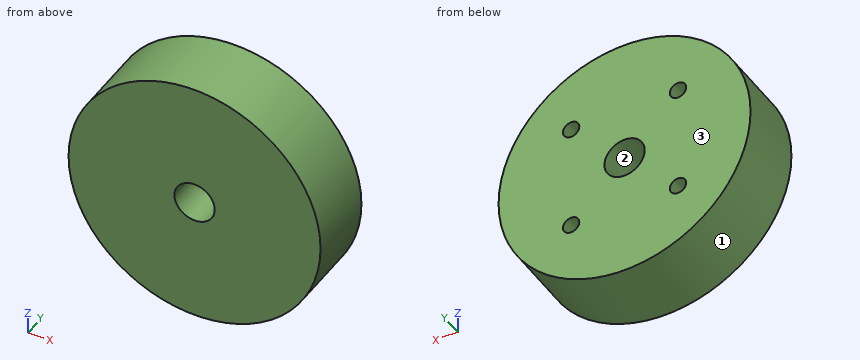
Autodesk Inventor part; units mm, degrees
ref_plane "YZ Plane" through (0, 0, 0) normal (1, 0, 0) x (0, 1, 0)
ref_plane "XZ Plane" through (0, 0, 0) normal (0, 1, 0) x (-1, 0, 0)
ref_plane "XY Plane" through (0, 0, 0) normal (0, 0, 1) x (1, 0, 0)
sketch "スケッチ5" plane through (0, 0, 0) normal (0, 1, 0) x (-1, 0, 0)
  circle A0 centre (0, 0) radius 25
  dimension "d23" = 50
extrude "押し出し2" add sketch "スケッチ5" along normal blind 14
sketch "スケッチ6" plane through (0, 14, 0) normal (0, 1, 0) x (1, 0, 0)
  circle A0 centre (0, 0) radius 4
  dimension "d26" = 8
extrude "押し出し3" cut sketch "スケッチ6" against normal blind 14
sketch "スケッチ7" plane through (0, 14, 0) normal (0, 1, 0) x (1, 0, 0)
  line L0 (0, 0) -> (10.6066, 10.6066)
  line L1 (0, 0) -> (15, 0) construction
  point P0 (-10.6066, 10.6066)
  point P1 (-10.6066, -10.6066)
  point P2 (10.6066, -10.6066)
  dimension "d29" = 15
  dimension "d30" = 45
  dimension "d33" = 360
hole "穴2" at (10.6066, 14, -10.6066) at (-10.6066, 14, -10.6066) at (-10.6066, 14, 10.6066) at (10.6066, 14, 10.6066) direction (0, -1, 0) diameter 3.242 depth 5 tip angle 118
properties part number "Stator" material "ステンレス鋼"
Read the model definition and answer for the solid it produces. Units are mm, in the model's axes. Face numbers are marked on the shaded views. Give positions to 0.01 mm unless a question says otherwise; leave off trailing zeros. Loops run counter-clockwise (first coordinate to the right, second up) from the corner with the lowest first, then second, coordinate; pieces in that order, holes last. Notation, with made-up numbers: (-33.5, -38.75) -> (-11.5, -38.75) arc R25 ccw to (-11.5, -5.75) -> close; hole circle Ø7 at (73, -10.5). An arc over 180 degrees is marked (long way). Use a Markdown table: item, result.
Q1. Section D-D, the plane y = 1 is taken. Determine the outline of the cut face in (x, z), then the cut area to 3 significant figures.
Solved:
| item | result |
|---|---|
| outline | circle Ø50 at (0, 0); hole circle Ø8 at (0, 0) |
| area | 1,910 mm^2 |
Q2. Find the intervals of material crossed by line 1 along Z through (x, y) = (0, 10.25); line 2 along X through (y, z) = (11.25, -9.5); line 3 along Z through (x, y) = (-2.5, 8.75), in increasing order.
Solved:
| item | result |
|---|---|
| line 1 | z = -25 to -4, 4 to 25 |
| line 2 | x = -23.12 to -11.79, -9.42 to 9.42, 11.79 to 23.12 |
| line 3 | z = -24.87 to -3.12, 3.12 to 24.87 |
Q3. Section A-A, the plane z = 0 is taken. Determine the outline of the cut face in (x, y).
Solved:
| item | result |
|---|---|
| outline | (-25, 0) -> (-4, 0) -> (-4, 14) -> (-25, 14) -> close; (4, 0) -> (25, 0) -> (25, 14) -> (4, 14) -> close |
Q4. Section C-C, the plane y = 13.25 is taken. Determine the outline of the cut face in (x, z).
Solved:
| item | result |
|---|---|
| outline | circle Ø50 at (0, 0); hole circle Ø3.24 at (-10.61, -10.61); hole circle Ø3.24 at (-10.61, 10.61); hole circle Ø8 at (0, 0); hole circle Ø3.24 at (10.61, -10.61); hole circle Ø3.24 at (10.61, 10.61) |
Q5. Section B-B, the plane x = 0 is taken. Determine the outline of the cut face in (y, z).
Solved:
| item | result |
|---|---|
| outline | (0, -25) -> (14, -25) -> (14, -4) -> (0, -4) -> close; (0, 4) -> (14, 4) -> (14, 25) -> (0, 25) -> close |
Q6. Determine the mould class of the marked faces 1, 2 and 3 for opening direction Z: pulls with the +Z half, pulls with the -Z half, needs draft (parallel to the pull), parting line crosses it, or undercut.
Solved:
| item | result |
|---|---|
| face 1 | parting line crosses it |
| face 2 | undercut |
| face 3 | needs draft |
Q7. Each of these flat-tipped pins is pushed along its axis until it touches: pin 1 (1 mm diameter, centred on y = 2.5, z = -3.5, fed in from -X); pin 2 (2 mm diameter, centred on y = 5, z = 4.5, fed in from +X); pin 3 (3 mm diameter, centred on x = -12, y = 3, fed in from -Z). Where does it stop, or does it pass through?
Solved:
| item | result |
|---|---|
| pin 1 | stops at x = -24.82 |
| pin 2 | stops at x = 24.75 |
| pin 3 | stops at z = -22.69 |
